Part model, mm, in its own coordinate system. A direction names the side the tool comes from. Coordinates: 2 decimals unless noted, no trailing zeros. Order: outer loops, then holes, each group sorted by start corner. A loop starts at its lowest first (then second) coordinate and runs counter-clockwise, first axis right, second up.
```python
from build123d import *

# Parameters (mm, degrees)
F0_W     = 698.5
F0_H     = 76.2
F1_DEPTH = 581.025
F2_W     = 660.4
F2_H     = 57.15
F3_DEPTH = 565.15


with BuildPart() as f1:
    # F0 (on Front) → F1 (new body)
    with BuildSketch(Plane.XZ):
        Polygon((0, 25.4), (0, 0), (361.95, 0), (1060.45, 0), (1422.4, 0), (1422.4, 25.4), align=None)
        with Locations((711.2, -38.1)):
            Rectangle(F0_W, F0_H)
    extrude(amount=F1_DEPTH)

    # F2 (on face) → F3 (cut)
    with BuildSketch(Plane.XZ.offset(581.025)):
        with Locations((711.2, -28.575)):
            Rectangle(F2_W, F2_H)
    extrude(amount=-F3_DEPTH, mode=Mode.SUBTRACT)


solid = f1.part
```
(1) Slice it at C-C, the plane x = 500. Give the cut face in (y, z) (3 decimals), then the cut area to 3 significant figures.
(2) Tool access for faces 1 (the face through (707, -15.875, -28)), 2 (the face through (361.95, -286, -39)), 3 (the face through (701, 0, -13)), 4 (the face through (0, -286, 13)), 5 (the face through (1060.45, -286, -39)): list every direction of +Z, -Z, +X, -X, +Y, -Y with a clear straight run to the whole face (end or side of a thin tool).
(3) Slice it at B-B, the plane z = -18. Give the cut face in (x, y) (3 decimals), then the cut area to 3 significant figures.
(4) Slice it at A-A, the plane y = -71. Give the cut face in (x, z).
(5) Probe line 1 (X direction, y = -305, z = -6); line 2 (Z direction, x = 560.5, y = -520); line 3 (Z direction, x = 1088.5, y = -371.5). List the from-to ranges inside material, lowest first.
(6) Pull direction X, two halves, no side cores. Call faces 6 (the face through (721, -286, 25.4)), 7 (the face through (381, -302, -29)), 8 (the face through (1422.4, -286, 13)): +X half, -X half, draft (parallel to the pull), parting line (faces both ways), or undercut.
(7) Drop flat-ended pins along their axis: pin 1 (3 mm diameter, centred on y = -358, z = -52.5, fed in from +X); pin 2 (6 mm diameter, centred on x = 250, y = -508, fed in from -Z); pin 3 (23 mm diameter, centred on y = -405, z = -31.5, fed in from -X). Give the stop position or say it passes through.
(8) Slice it at D-D, the plane x = 185.5. Give the cut face in (y, z) (3 decimals), then the cut area to 3 significant figures.
Here are the results:
1. outline: (-581.025, -76.2) - (0, -76.2) - (0, 25.4) - (-581.025, 25.4) - (-581.025, 0) - (-15.875, 0) - (-15.875, -57.15) - (-581.025, -57.15) - close
1. area: 26,700 mm2
2. face 1: -Y
2. face 2: -Z, -X, +Y, -Y
2. face 3: +Z, -Z, +X, -X, +Y
2. face 4: +Z, -Z, -X, +Y, -Y
2. face 5: -Z, +X, +Y, -Y
3. outline: (361.95, -581.025) - (381, -581.025) - (381, -15.875) - (1041.4, -15.875) - (1041.4, -581.025) - (1060.45, -581.025) - (1060.45, 0) - (361.95, 0) - close
3. area: 32,600 mm2
4. outline: (0, 0) - (361.95, 0) - (361.95, -76.2) - (1060.45, -76.2) - (1060.45, 0) - (1422.4, 0) - (1422.4, 25.4) - (0, 25.4) - close; hole (381, -57.15) - (1041.4, -57.15) - (1041.4, 0) - (381, 0) - close
5. line 1: x = 361.95 to 381, 1041.4 to 1060.45
5. line 2: z = -76.2 to -57.15, 0 to 25.4
5. line 3: z = 0 to 25.4
6. face 6: draft
6. face 7: undercut
6. face 8: +X half
7. pin 1: stops at x = 1060.45
7. pin 2: stops at z = 0
7. pin 3: stops at x = 361.95
8. outline: (-581.025, 0) - (0, 0) - (0, 25.4) - (-581.025, 25.4) - close
8. area: 14,800 mm2
